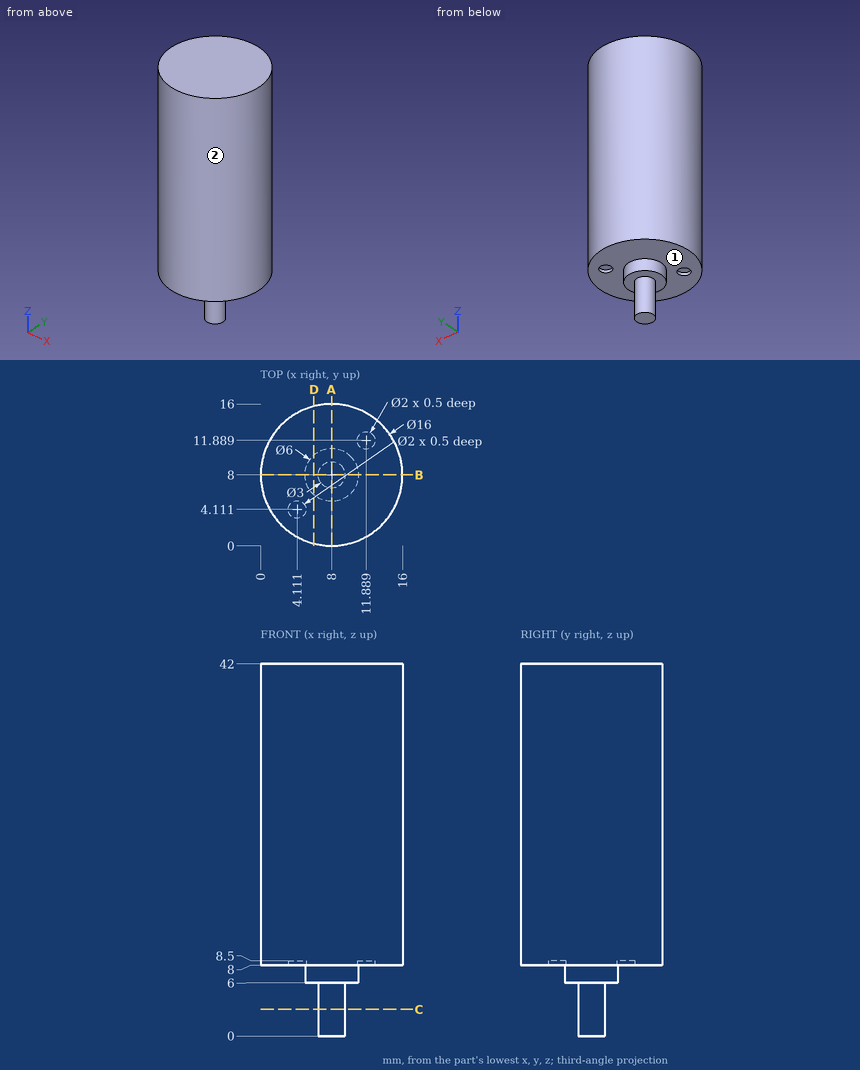
Job drawing, mm, ordinate dimensions from the low corner. One solid piece. A direction names the side the tool comes from. Give positions to 0.01 mm unless a question says otherwise; leave off trailing zeros. Loops run counter-clockwise (first coordinate to the right, second up) from the corner with the lowest first, then second, coordinate; pieces in that order, holes last. Notation, with made-up numbers: (-31, -8.5) - (5, -8.5) arc R14 ccw to (5, 15.5) - close; hole circle Ø7 at (20, 70). An arc over 180 degrees is marked (long way). Use one line per item in the form item = value.
(1) Cut at A-A (x = 8). Give the cut face in (y, z).
Determined:
outline = (0, 8) - (5, 8) - (5, 6) - (6.5, 6) - (6.5, 0) - (9.5, 0) - (9.5, 6) - (11, 6) - (11, 8) - (16, 8) - (16, 42) - (0, 42) - close
(2) 3-axis set-ups, long thin cutter, end or side, ignore diameter. For the marked faces 1 and 2: which of +Z, -Z, +X, -X, +Y, -Y reach the whole face in a straight line?
Determined:
face_1 = -Z
face_2 = +Z, -Z
(3) Drill centre lines: L1, parallel to Z at x = 8.5, y = 5.25; L2, parallel to Z at x = 4.5, y = 8; L3, parallel to Y at x = 13, z = 39.5 (3 decimals). Where is each one in solid material? Low to high.
Determined:
L1 = 6 to 42
L2 = 8 to 42
L3 = 1.755 to 14.245
(4) Cut at D-D (x = 6). Give the cut face in (y, z).
Determined:
outline = (0.25, 8) - (5.76, 8) - (5.76, 6) - (10.24, 6) - (10.24, 8) - (15.75, 8) - (15.75, 42) - (0.25, 42) - close
(5) Cut at C-C (z = 3). Give the cut face in (x, y), then the cut area to 3 significant figures.
Determined:
outline = circle Ø3 at (8, 8)
area = 7.07 mm^2
(6) Drop flat-ended pins along their axis: P1, Ø3, axis at x = 8.5, y = 7, coming from the -Z side; P2, Ø1, axis at x = 11, y = 14, coming from the -Z side; P3, Ø0.6, axis at x = 4, y = 4.5, coming from the -Z side; P4, Ø1, axis at x = 5.5, y = 8.5, coming from the -Z side. Give the stop position or say it passes through.
Determined:
P1 = 0
P2 = 8
P3 = 8.5
P4 = 6
